Autodesk Inventor part; units mm, degrees
ref_plane "YZ Plane" through (0, 0, 0) normal (1, 0, 0) x (0, 1, 0)
ref_plane "XZ Plane" through (0, 0, 0) normal (0, 1, 0) x (-1, 0, 0)
ref_plane "XY Plane" through (0, 0, 0) normal (0, 0, 1) x (1, 0, 0)
sketch "Sketch1" plane through (0, 0, 0) normal (0, 1, 0) x (-1, 0, 0)
  line L0 (0, 0) -> (50, 0)
  line L1 (50, 0) -> (50, -32)
  line L2 (50, -32) -> (0, -32)
  line L3 (0, -32) -> (0, 0)
  line L4 (0, -27.752) -> (5.747, -27.752)
  circle A0 centre (5.747, -27.752) radius 1.25
  line L5 (25, 0) -> (25, -16) construction
  line L6 (25, -16) -> (0, -16) construction
  circle A1 centre (5.747, -4.248) radius 1.25
  circle A2 centre (44.253, -27.752) radius 1.25
  circle A3 centre (44.253, -4.248) radius 1.25
  circle A4 centre (25, -16) radius 3.75
  dimension "d0" = 50
  dimension "d1" = 32
  dimension "d2" = 5.747
  dimension "d3" = 4.248
  dimension "d4" = 2.5
  dimension "d5" = 7.5
extrude "Extrusion1" add sketch "Sketch1" along normal blind 4
sketch "Sketch2" plane through (0, 4, 0) normal (0, 1, 0) x (1, 0, 0)
  circle A0 centre (-25, 16) radius 3.75
  circle A1 centre (-25, 16) radius 12
  line L0 (-25, 16) -> (-32, 16)
  line L1 (-25, 16) -> (-18, 16)
  circle A2 centre (-32, 16) radius 0.75
  circle A3 centre (-18, 16) radius 0.75
  point P0 (0, 0)
  dimension "d8" = 24
  dimension "d9" = 7
  dimension "d10" = 7
  dimension "d11" = 1.5
  dimension "d12" = 1.5
extrude "Extrusion2" add sketch "Sketch2" along normal blind 2.325
sketch "Sketch3" plane through (-25, 6.325, -16) normal (0, 1, 0) x (1, 0, 0)
  circle A0 centre (0, 0) radius 12
  circle A1 centre (0, 0) radius 3.75
  circle A2 centre (-7, 0) radius 0.75
  circle A3 centre (7, 0) radius 0.75
  line L0 (-7, 0) -> (-7.5625, 0)
  line L1 (-7, 0) -> (-7, -2.877)
  line L2 (-7, 0) -> (-10.333, 0)
  line L3 (-10.333, 2.1388) -> (-10.333, 2.277)
  line L4 (-10.333, -2.1388) -> (-10.333, -2.277)
  line L5 (-10.333, -2.1388) -> (-10.005, -2.1388)
  line L6 (-10.333, -2.1388) -> (-2.5151, -2.7815)
  line L7 (-10.333, -2.1388) -> (-2.4887, -2.1388) construction
  line L8 (0, 0) -> (0, 2.5608)
  line L9 (-10.333, 2.1388) -> (-2.5151, 2.7815)
  arc A4 (-5.1785, -2.5625) -> (-4.792, -2.1388) centre (-7.5625, 0) ccw
  arc A5 (-10.333, 2.1388) -> (-10.333, -2.1388) centre (-7.5625, 0) ccw
  line L10 (10.333, -2.1388) -> (2.5151, -2.7815)
  line L11 (10.333, 2.1388) -> (2.5151, 2.7815)
  arc A6 (10.333, -2.1388) -> (10.333, 2.1388) centre (7.5625, 0) ccw
  arc A7 (-3.0803, -2.1388) -> (2.5151, -2.7815) centre (0, 0) ccw
  arc A8 (2.5151, 2.7815) -> (-2.5151, 2.7815) centre (0, 0) ccw
  point P0 (25, -16)
  dimension "d15" = 0.5625
  dimension "d17" = 2.877
  dimension "d18" = 3.333
  dimension "d20" = 2.277
  dimension "d21" = 4.7
extrude "Extrusion3" add sketch "Sketch3" along normal blind 3.675 contours A0
properties part number "base"
Geometry: final body of the model. Coordinates: model frame, mm. A direction names the side the tool comes from. Give positions to 0.01 mm unless a question says otherwise; leave off trailing zeros. Loops run counter-clockwise (first coordinate to the right, second up) from the corner with the lowest first, then second, coordinate; pieces in that order, holes last. Notation, with made-up numbers: (79, -17.5) -> (104, -17.5) arc R13 cw to (104, -0.5) -> close; hole circle Ø2 at (63.25, 18). An arc over 180 degrees is marked (long way). Put each result on its own line as item: value.
1. Pin query (flat end, axial travel): P1, Ø8, axis at x = -20.5, z = -17.5, coming from the +Y side; P2, Ø3, axis at x = -44.253, z = -4.248, coming from the +Y side; P3, Ø2, axis at y = 5.5, z = -14, coming from the +X side; P4, Ø3, axis at x = -18.5, z = -16.5, coming from the +Y side (3 decimals). Return the tip coordinate at first contact, or that it passes through.
Taken from the geometry:
P1: stops at y = 10
P2: stops at y = 4
P3: stops at x = -13.04
P4: stops at y = 6.325
2. Set-up query: faces 5 (the flat face through (-25, 0, -12)), 6 (the flat face through (-19, 6.325, -16)). Return all of +Z, -Z, +X, -X, +Y, -Y with unobstructed straight access to the full face (end or side cutting, diameter ignored); none if empty.
Taken from the geometry:
face 5: +Z, -Z, +X, -X, -Y
face 6: +Y
3. Cut plane A-A (y = 9). Return the cut outline in (x, z).
Taken from the geometry:
outline: circle Ø24 at (-25, -16); hole (-35.33, -18.14) -> (-27.52, -18.78) arc R3.75 ccw to (-22.48, -18.78) -> (-14.67, -18.14) arc R3.5 ccw to (-14.67, -13.86) -> (-22.48, -13.22) arc R3.75 ccw to (-27.52, -13.22) -> (-35.33, -13.86) arc R3.5 ccw to start
4. Cut plane D-D (y = 4.5). Return the cut outline in (x, z), plus the area to 3 significant figures.
Taken from the geometry:
outline: circle Ø24 at (-25, -16); hole circle Ø1.5 at (-32, -16); hole circle Ø7.5 at (-25, -16); hole circle Ø1.5 at (-18, -16)
area: 405 mm2
5. Pull-direction query (X, two-part tool) for faces 1 (the cylindrical face through (-13.554, 6.958, -12.396)), 2 (the cylindrical face through (-6.324, 1.972, -3.139)), 3 (the flat face through (-50, 2, -16)), 4 (the flat face through (-28, 10, -19)); classes: released by +X, released by -X, zero draft, split by the parting line, or undercut.
Taken from the geometry:
face 1: split by the parting line
face 2: undercut
face 3: released by -X
face 4: zero draft
6. Ray query, line 1 along X through (y, z) = (5.8, -16); line 2 along X through (y, z) = (2, -16); line 3 along Z through (x, y) = (-25, 4.75). Return the intervals inside material, ascending. Write a range as [from, to].
Taken from the geometry:
line 1: x = [-37, -32.75], [-31.25, -28.75], [-21.25, -18.75], [-17.25, -13]
line 2: x = [-50, -28.75], [-21.25, 0]
line 3: z = [-28, -19.75], [-12.25, -4]
7. Cut plane C-C (z = -16). Return the cut outline in (x, y) (3 decimals).
Taken from the geometry:
outline: (-50, 0) -> (-28.75, 0) -> (-28.75, 6.325) -> (-31.25, 6.325) -> (-31.25, 4) -> (-32.75, 4) -> (-32.75, 6.325) -> (-36.063, 6.325) -> (-36.063, 10) -> (-37, 10) -> (-37, 4) -> (-50, 4) -> close; (-21.25, 0) -> (0, 0) -> (0, 4) -> (-13, 4) -> (-13, 10) -> (-13.937, 10) -> (-13.937, 6.325) -> (-17.25, 6.325) -> (-17.25, 4) -> (-18.75, 4) -> (-18.75, 6.325) -> (-21.25, 6.325) -> close
8. Cut plane B-B (x = -25). Return the cut outline in (y, z).
Taken from the geometry:
outline: (0, -32) -> (4, -32) -> (4, -28) -> (10, -28) -> (10, -19.75) -> (0, -19.75) -> close; (0, -12.25) -> (10, -12.25) -> (10, -4) -> (4, -4) -> (4, 0) -> (0, 0) -> close
